Answer from the drawing. Dimensions are ordinates in mm from the lowest x, y and z of the part. A direction names the side the tool comes from. Coordinates: 2 decimals unless noted, no trailing zeros. Loops run counter-clockwise (first coordinate to the right, second up) from the corner with the lowest first, then second, coordinate; pieces in that order, holes last. Notation, with made-up numbers: M -27.75,9.25 L 30.25,9.25 A35 ccw 30.25,41.25 Z; hole C 2,35.5 d6. An arc over 180 degrees is marked long. Put each result on its own line as item: value.
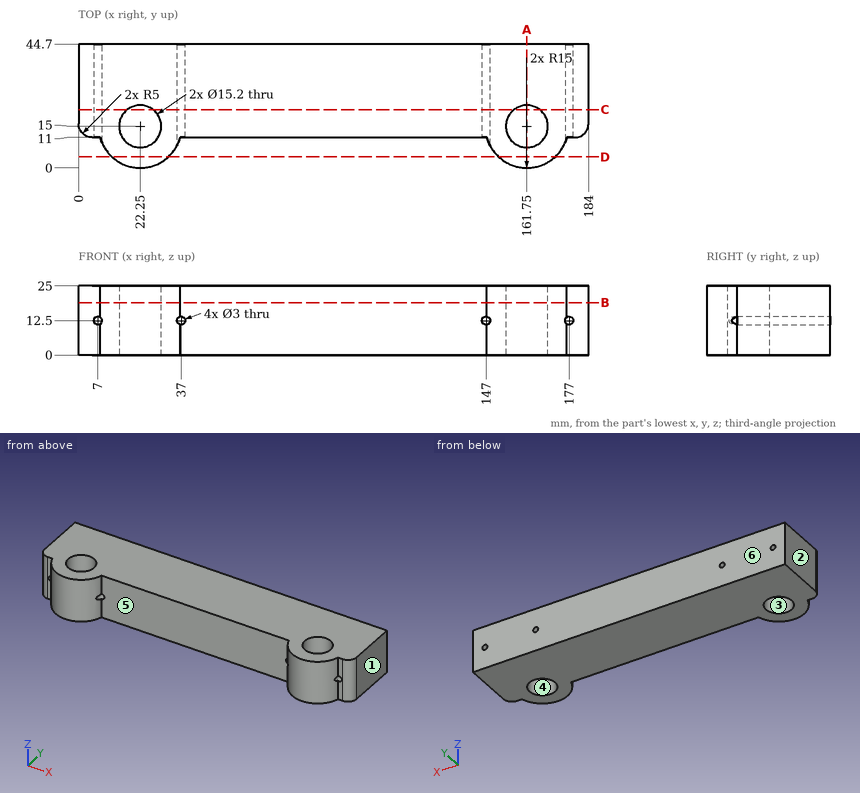
1) Find section B-B, the plane z = 19. Write down the section's boundary in (x, y).
Answer list:
outline: M 0,16 A5 ccw 5,11 L 7.79,11 A15 ccw 36.71,11 L 147.29,11 A15 ccw 176.21,11 L 179,11 A5 ccw 184,16 L 184,44.7 L 0,44.7 Z; hole C 22.25,15 d15.2; hole C 161.75,15 d15.2
2) Find section A-A, the plane x = 161.75. Write down the section's boundary in (y, z).
Answer list:
outline: M 0,0 L 7.4,0 L 7.4,25 L 0,25 Z; M 22.6,0 L 44.7,0 L 44.7,25 L 22.6,25 Z
3) Straight lines are drawn through the part: line 1 (Z direction, x = 147, y = 20.5); line 2 (Y direction, x = 161.75, z = 6); line 3 (X direction, y = 14, z = 24.25). For each, find the intervals that lie inside material, in ascending order. Write a range as [from, to].
Answer list:
line 1: z = [0, 11], [14, 25]
line 2: y = [0, 7.4], [22.6, 44.7]
line 3: x = [0.42, 14.72], [29.78, 154.22], [169.28, 183.58]
4) Determine the mould class of the marked faces 1, 2, 3 and 4 for opening direction X: released by +X, released by -X, zero draft, split by the parting line, or undercut.
Answer list:
face 1: released by +X
face 2: released by -X
face 3: undercut
face 4: undercut
5) Which of the six approach directions +Z, -Z, +X, -X, +Y, -Y give full straight-line access (tool end or side, diameter ignored) to the marked faces 5 and 6?
Answer list:
face 5: +Z, -Z, -Y
face 6: +Z, -Z, +X, -X, +Y
6) Given pin 1 Ø3.5 at (x, z) = (177, 12.5) entering from +Y; pin 2 Ø2 at (x, z) = (124, 16) entering from -Y; pin 3 Ø3 at (x, z) = (148.5, 18.5) entering from -Y, each flat-ended and moving along its own axis, determine where each tip first touches the part or whether it passes through.
Answer list:
pin 1: stops at y = 44.7
pin 2: stops at y = 11
pin 3: stops at y = 5.68
7) Find section D-D, the plane y = 4. Write down the section's boundary in (x, z).
Answer list:
outline: M 12.05,0 L 32.45,0 L 32.45,25 L 12.05,25 Z; M 151.55,0 L 171.95,0 L 171.95,25 L 151.55,25 Z
8) Find section C-C, the plane y = 21. Write down the section's boundary in (x, z), plus the area to 3 significant figures.
Answer list:
outline: M 0,0 L 17.59,0 L 17.59,25 L 0,25 Z; M 26.91,0 L 157.09,0 L 157.09,25 L 26.91,25 Z; M 166.41,0 L 184,0 L 184,25 L 166.41,25 Z; hole C 7,12.5 d3; hole C 37,12.5 d3; hole C 147,12.5 d3; hole C 177,12.5 d3
area: 4,110 mm^2
